from build123d import *

# Parameters (mm, degrees)
ESQUISSE1_R             = 15
BOSS_EXTRU_1_DEPTH      = 11.5
ESQUISSE2_OUTSIDE_W     = 40.792
ESQUISSE2_OUTSIDE_H     = 40.792
ESQUISSE2_OUTSIDE_R     = 11.5
ENL_V_MAT_EXTRU_1_DEPTH = 10
ENL_V_MAT_EXTRU_2_REACH = 26.13
ESQUISSE3_R             = 10
CONG_1_R                = 1
CONG_2_R                = 1
ENL_V_MAT_EXTRU_3_DEPTH = 25.12985702402731
CHANFREIN1_SIZE         = 0.5


with BuildPart() as part:
    # Esquisse1 → Boss.-Extru.1 (new body)
    with BuildSketch(Plane.XY):
        Circle(ESQUISSE1_R)
    extrude(amount=BOSS_EXTRU_1_DEPTH)

    # Esquisse2 outside → Enlèv. mat.-Extru.1 (cut)
    with BuildSketch(Plane.XY.offset(11.5)):
        Rectangle(ESQUISSE2_OUTSIDE_W, ESQUISSE2_OUTSIDE_H)
        Circle(ESQUISSE2_OUTSIDE_R, mode=Mode.SUBTRACT)
    extrude(amount=-ENL_V_MAT_EXTRU_1_DEPTH, mode=Mode.SUBTRACT)

    # Esquisse3 → Enlèv. mat.-Extru.2 (cut, up to next)
    with BuildSketch(Plane.XY.offset(11.5), mode=Mode.PRIVATE) as enl_v_mat_extru_2_sk1:
        Circle(ESQUISSE3_R)
    enl_v_mat_extru_2_tool1 = extrude(enl_v_mat_extru_2_sk1.sketch, amount=-ENL_V_MAT_EXTRU_2_REACH, mode=Mode.PRIVATE) & part.part
    add(enl_v_mat_extru_2_tool1.solids().sort_by_distance((0, 0, 11.5))[0], mode=Mode.SUBTRACT)

    # Congé1
    cong_1_edges = [part.edges().sort_by_distance(p)[0] for p in [
        (-11.5, 1.41e-15, 1.5),
    ]]
    fillet(cong_1_edges, radius=CONG_1_R)

    # Congé2
    cong_2_edges = [part.edges().sort_by_distance(p)[0] for p in [
        (-10, 1.22e-15, 0),
    ]]
    fillet(cong_2_edges, radius=CONG_2_R)

    # Esquisse4 → Enlèv. mat.-Extru.3 (cut, through all)
    with BuildSketch(Plane.XY.offset(11.5)):
        Polygon((0.5, 9), (-0.5, 9), (-0.5, 10.988630487917954), (-2.0000000000000004, 15), (2, 15), (0.5, 10.988630487917954), align=None)
    extrude(amount=-ENL_V_MAT_EXTRU_3_DEPTH, mode=Mode.SUBTRACT)

    # Chanfrein1
    chanfrein1_edges = [part.edges().sort_by_distance(p)[0] for p in [
        (-7.886330667871463, -8.36993360768113, 11.5),
    ]]
    chamfer(chanfrein1_edges, length=CHANFREIN1_SIZE)


solid = part.part
CAD build for the part. Positions are in the model's coordinates, mm. A direction names the side the tool comes from. Round coordinates to 2 decimals unless told otherwise and drop trailing zeros. Write each loop counter-clockwise with the first axis right and the second up, starting at its lowest first coordinate (ties: lowest second). Pieces come first, ordered by that corner, then holes. Notation, with made-up numbers: M 56,64.25 L 114,64.25 A10 ccw 114,79.25 Z; hole C 53.5,61.25 d8. An arc over 180 degrees is marked long. Use a Markdown table: item, result. Add a question column.
1. Slice it at C-C on x = -13. Give the cut face in (y, z).
2. Slice it at B-B on z = 7.5. Give the cut face in (x, y), then the cut area to 3 significant figures.
3. Drill centre lines: probe 1 along X at (y, z) = (0, 7); probe 2 along Y at (x, z) = (0, 8.75); probe 3 along X at (y, z) = (-8.25, 8). Where is each one in solid material? Low to high.
4. Flat gauge pins, fed straight in: P1, Ø2, axis at y = 8, z = 9.5, coming from the -X side; P2, Ø3, axis at y = 1, z = 8, coming from the -X side; P3, Ø6, axis at x = 11.5, z = 5.5, coming from the +Y side. Where does each tip first touch, or does it go through?
5. 3-axis set-ups, long thin cutter, end or side, ignore diameter. For faces 1 (the face through (0.584, 11.213, 3.221)), 2 (the face through (-9, -9, 1.5)), 3 (the face through (-9, -7, 0)): which of +Z, -Z, +X, -X, +Y, -Y reach the whole face in a straight line?
6. Pull direction X, two halves, no side cores. Call faces 4 (the face through (-0.5, 10.5, 5.8)), 5 (the face through (-10, -2, 11.5)), 6 (the face through (-0.632, -14.987, 0.74)): released by +X, released by -X, zero draft, split by the parting line, or undercut.
7. Slice it at A-A on x = 0. Give the cut face in (y, z), then the cut area to 3 significant figures.
Reply:
| question | item | result |
|---|---|---|
| 1 | outline | M -7.48,0 L 7.48,0 L 7.48,1.5 L -7.48,1.5 Z |
| 2 | outline | M -0.68,11.48 A11.5 ccw long 0.68,11.48 L 0.5,10.99 L 0.5,9.99 A10 cw long -0.5,9.99 L -0.5,10.99 Z |
| 2 | area | 99.7 mm^2 |
| 3 | probe 1 | x = -11.5 to -10, 10 to 11.5 |
| 3 | probe 2 | y = -11.5 to -10 |
| 3 | probe 3 | x = -8.01 to -5.65, 5.65 to 8.01 |
| 4 | P1 | stops at x = -9.12 |
| 4 | P2 | stops at x = -11.5 |
| 4 | P3 | stops at y = 7.75 |
| 5 | face 1 | +Z, -Z, +Y |
| 5 | face 2 | +Z |
| 5 | face 3 | -Z, +X, -X, +Y, -Y |
| 6 | face 4 | undercut |
| 6 | face 5 | zero draft |
| 6 | face 6 | split by the parting line |
| 7 | outline | M -15,0 L -11,0 A1 ccw -10,1 L -10,11.5 L -11,11.5 L -11.5,11 L -11.5,2.5 A1 cw -12.5,1.5 L -15,1.5 Z |
| 7 | area | 22.4 mm^2 |
